Source: CAD feature listing. Evaluate the final solid. Frame: model axes, mm. A direction names the side the tool comes from. Round coordinates to 2 decimals unless told otherwise and drop trailing zeros. Order: outer loops, then holes, each group sorted by start corner. A loop starts at its lowest first (then second) coordinate and runs counter-clockwise, first axis right, second up. Notation, with made-up numbers: (6.25, 4) -> (22.25, 4) arc R17 ccw to (22.25, 37) -> close; hole circle Ø8 at (10.5, 33.25). An arc over 180 degrees is marked (long way). One line per item, written item: value. Start each with the question number.
1) Ray query, L1, parallel to Z at x = -1.75, y = 3.5; L2, parallel to Y at x = -6.5, z = -0.55; L3, parallel to Z at x = -0.95, y = 3.5. Return the intervals inside material, ascending.
2) Pin query (flat end, axial travel): P1, Ø3, axis at y = 5, z = -3.5, coming from the -X side; P2, Ø1.5, axis at y = 4, z = -4, coming from the +X side; P3, Ø3.5, axis at x = -5.5, y = 4, coming from the -Z side. Return the tip coordinate at first contact, or that it passes through.
3) Section D-D (y = 0.75). Return the cut outline in (x, z), and give its area (3 significant figures).
4) Section A-A (z = -6). Return the cut outline in (x, y).
5) Section C-C (x = -6.5). Return the cut outline in (y, z), and give its area (3 significant figures).
6) Reachability of faces 1 (the face through (-0.986, 4.248, -6.976)), 2 (the face through (-1, 6, -5)) from +Z, -Z, +X, -X, +Y, -Y: full face, straight path, thin tool, end or side. Return the list, or none.
7) Mould query, pull axis Z, two halves, no side actions, for faces 3 (the face through (-2, 2, -6)), 4 (the face through (-0.5, 3.5, -11)), 5 (the face through (-4.9, 2.7, 0)), 6 (the face through (-1.7, 4.7, -7.6)). Classes: pulls with the +Z half, pulls with the -Z half, needs draft (parallel to the pull), parting line crosses it, or undercut.
8) Section B-B (y = 3.5). Return the cut outline in (x, z).
Autodesk Inventor part; units mm, degrees
ref_plane "YZ Plane" through (0, 0, 0) normal (1, 0, 0) x (0, 1, 0)
ref_plane "XZ Plane" through (0, 0, 0) normal (0, 1, 0) x (-1, 0, 0)
ref_plane "XY Plane" through (0, 0, 0) normal (0, 0, 1) x (1, 0, 0)
sketch "Sketch1" plane through (0, 0, 0) normal (0, 1, 0) x (-1, 0, 0)
  line L0 (1, -11) -> (0, -11)
  line L1 (0, -11) -> (0, 0)
  line L2 (0, 0) -> (10, 0)
  line L3 (10, 0) -> (10, -1)
  line L4 (9, -1) -> (1, -1)
  line L5 (1, -1) -> (1, -10)
  line L6 (1, -10) -> (1, -11)
  line L7 (9, -1) -> (10, -1)
  dimension "d0" = 10
  dimension "d1" = 11
  dimension "d2" = 1
extrude "Extrusion1" add sketch "Sketch1" along normal blind 7
sketch "Sketch2" plane through (-10, 0, 0) normal (0, 0, 1) x (1, 0, 0)
  line L0 (-7.7219, 3.5) -> (14.6275, 3.5)
  line L1 (3.5, 11.0535) -> (3.5, -3.5767)
  line L2 (10, 0) -> (10, 7)
  line L3 (0, 0) -> (0, 7)
  point P0 (10, 3.5)
  point P1 (3.5, 3.5)
  dimension "d13" = 6.5
hole "Hole1" at (-6.5, 3.5, 0) direction (0, 0, -1) diameter 3.2 end through all
sketch "Sketch3" plane through (-1, 0, -11) normal (-1, 0, 0) x (0, 0, 1)
  line L0 (5, -6.7291) -> (5, 15.8224)
  line L1 (-2.4783, 3.5) -> (17.6078, 3.5)
  line L2 (0, 0) -> (10, 0)
  line L3 (10, 0) -> (10, 7)
  line L4 (0, 7) -> (10, 7)
  line L5 (0, 0) -> (0, 7)
  line L6 (11, 0) -> (11, 7)
  circle A0 centre (5, 3.5) radius 2
  point P0 (0, 3.5)
  dimension "d14" = 6
  dimension "d15" = 4
extrude "Extrusion2" add sketch "Sketch3" along normal blind 1 contours A0 L1 L0 | L0 L1 A0 | L1 A0 L0 | L0 A0 L1
fillet "Fillet1" radius 0.4 1 edges at (-1, 3.5, -8)
sketch "Sketch4" plane through (-2, 3.5, -6) normal (-1, 0, 0) x (0, 0, 1)
  point P0 (6, -3.5)
  point P1 (0, 0)
hole "Hole2" at (-2, 3.5, -6) direction (1, 0, 0) diameter 2.459 end through all
properties part number "Single Thrd Right Support Farnell1466883"
Findings:
1. L1: -8 to -7.23, -4.77 to -4, -1 to 0
1. L2: 0 to 1.9, 5.1 to 7
1. L3: -11 to -7.23, -4.77 to 0
2. P1: x = -2
2. P2: x = 0
2. P3: z = -1
3. outline: (-10, -1) -> (-1, -1) -> (-1, -11) -> (0, -11) -> (0, 0) -> (-10, 0) -> close
3. area: 20.0 mm2
4. outline: (-2, 1.5) -> (-1.4, 1.5) arc R0.4 cw to (-1, 1.1) -> (-1, 0) -> (0, 0) -> (0, 2.27) -> (-2, 2.27) -> close; (-2, 4.73) -> (0, 4.73) -> (0, 7) -> (-1, 7) -> (-1, 5.9) arc R0.4 cw to (-1.4, 5.5) -> (-2, 5.5) -> close
5. outline: (0, -1) -> (1.9, -1) -> (1.9, 0) -> (0, 0) -> close; (5.1, -1) -> (7, -1) -> (7, 0) -> (5.1, 0) -> close
5. area: 3.80 mm2
6. face 1: +X, -X
6. face 2: -X
7. face 3: needs draft
7. face 4: pulls with the -Z half
7. face 5: pulls with the +Z half
7. face 6: undercut
8. outline: (-10, -1) -> (-8.1, -1) -> (-8.1, 0) -> (-10, 0) -> close; (-4.9, -1) -> (-1, -1) -> (-1, -3.6) arc R0.4 cw to (-1.4, -4) -> (-2, -4) -> (-2, -4.77) -> (0, -4.77) -> (0, 0) -> (-4.9, 0) -> close; (-2, -8) -> (-1.4, -8) arc R0.4 cw to (-1, -8.4) -> (-1, -11) -> (0, -11) -> (0, -7.23) -> (-2, -7.23) -> close
